```python
from build123d import *

# Parameters (mm, degrees)
ESQUISSE1_W             = 42
ESQUISSE1_H             = 42
BOSS_EXTRU_1_DEPTH      = 34
ESQUISSE2_R             = 11
BOSS_EXTRU_2_DEPTH      = 2
ESQUISSE3_R             = 2.5
BOSS_EXTRU_3_DEPTH      = 11.5
CHANFREIN1_SIZE         = 4
ESQUISSE4_W             = 17
ESQUISSE4_H             = 10
BOSS_EXTRU_4_DEPTH      = 5
ESQUISSE5_R             = 1.5
ENL_V_MAT_EXTRU_1_DEPTH = 5


with BuildPart() as part:
    # Esquisse1 → Boss.-Extru.1 (new body)
    with BuildSketch(Plane.XY):
        with Locations((21, 21)):
            Rectangle(ESQUISSE1_W, ESQUISSE1_H)
    extrude(amount=BOSS_EXTRU_1_DEPTH)

    # Esquisse2 → Boss.-Extru.2 (add)
    with BuildSketch(Plane.XY.offset(34)):
        with Locations((21, 21)):
            Circle(ESQUISSE2_R)
    extrude(amount=BOSS_EXTRU_2_DEPTH)

    # Esquisse3 → Boss.-Extru.3 (add)
    with BuildSketch(Plane.XY.offset(36)):
        with Locations((21, 21)):
            Circle(ESQUISSE3_R)
    extrude(amount=BOSS_EXTRU_3_DEPTH)

    # Chanfrein1
    chanfrein1_edges = [part.edges().sort_by_distance(p)[0] for p in [
        (0, 42, 17),
        (42, 42, 17),
        (42, 0, 17),
        (0, 0, 17),
    ]]
    chamfer(chanfrein1_edges, length=CHANFREIN1_SIZE)

    # Esquisse4 → Boss.-Extru.4 (add)
    with BuildSketch(Plane(origin=(0, 42, 0), x_dir=(1, 0, 0), z_dir=(0, 1, 0))):
        with Locations((21, -5)):
            Rectangle(ESQUISSE4_W, ESQUISSE4_H)
    extrude(amount=BOSS_EXTRU_4_DEPTH)

    # Esquisse5 → Enlèv. mat.-Extru.1 (cut)
    with BuildSketch(Plane.XY.offset(34)):
        with Locations((5.5, 36.5)):
            Circle(ESQUISSE5_R)
        with Locations((36.5, 36.5)):
            Circle(ESQUISSE5_R)
        with Locations((36.5, 5.5)):
            Circle(ESQUISSE5_R)
        with Locations((5.5, 5.5)):
            Circle(ESQUISSE5_R)
    extrude(amount=-ENL_V_MAT_EXTRU_1_DEPTH, mode=Mode.SUBTRACT)


solid = part.part
```
Design review of the part built by this model. Coordinates are the model's own, in mm. A direction names the side the tool comes from. Coordinates: 2 decimals unless noted, no trailing zeros. Loops run counter-clockwise (first coordinate to the right, second up) from the corner with the lowest first, then second, coordinate; pieces in that order, holes last. Notation, with made-up numbers: (-29, 5) - (12, 5) arc R15 ccw to (12, 27) - close; hole circle Ø3 at (-31, 73.5). An arc over 180 degrees is marked (long way). Use CSV: the item, a comma, the result in double quotes. Start each with the question number.
1) Consider section A-A on x = 21. Write out the cut boundary in (y, z), then the cut area to 3 significant figures.
2) Consider section D-D on y = 36.5. Write out the cut boundary in (x, z), then the cut area to 3 significant figures.
3) Tool access review of faces 1 (the flat face through (12.5, 44, 5)), 2 (the cylindrical face through (4.3, 4.6, 31.5)), 3 (the flat face through (29.5, 44, 5)), 4 (the flat face through (21, 44, 10)): name each direction out of +Z, -Z, +X, -X, +Y, -Y from which nothing blocks a thin tool from reaching the whole face with its end or side.
4) Consider section C-C on z = 28. Write out the cut boundary in (x, y), then the cut area to 3 significant figures.
5) Consider section B-B on y = 21. Write out the cut boundary in (x, z).
6) The part is to be moulded in two halves that separate along Y. For faces 5 (the flat face through (2, 2, 17)), 6 (the flat face through (36, 37, 29)), 7 (the flat face through (2, 40, 17)), 8 (the flat face through (5, 37, 29)), say which applies: +Y half, -Y half, draft (parallel to the pull), parting line (faces both ways), or undercut.
7) Wall thickness on L1, parallel to Y at x = 36.5, z = 30.6; L2, parallel to Y at x = 5, z = 31: over which ranges is each line inside the solid? List them lowest first. Write a range as from..to.
8) For pin 1 Ø3.5 at (x, y) = (5.5, 37) entering from +Z; pin 2 Ø1 at (x, y) = (16.5, 16) entering from +Z; pin 3 Ø2.5 at (y, z) = (45.5, 3) entering from -X, all flat-tipped, find the tip position at first contact; note any pin that passes through.
Geometry says:
1,outline,"(0, 0) - (47, 0) - (47, 10) - (42, 10) - (42, 34) - (32, 34) - (32, 36) - (23.5, 36) - (23.5, 47.5) - (18.5, 47.5) - (18.5, 36) - (10, 36) - (10, 34) - (0, 34) - close"
1,area,"1,580 mm^2"
2,outline,"(0, 0) - (42, 0) - (42, 34) - (38, 34) - (38, 29) - (35, 29) - (35, 34) - (7, 34) - (7, 29) - (4, 29) - (4, 34) - (0, 34) - close"
2,area,"1,400 mm^2"
3,face 1,"+Z, -Z, -X, +Y"
3,face 2,"+Z"
3,face 3,"+Z, -Z, +X, +Y"
3,face 4,"+Z, +X, -X, +Y"
4,outline,"(0, 4) - (4, 0) - (38, 0) - (42, 4) - (42, 38) - (38, 42) - (4, 42) - (0, 38) - close"
4,area,"1,730 mm^2"
5,outline,"(0, 0) - (42, 0) - (42, 34) - (32, 34) - (32, 36) - (23.5, 36) - (23.5, 47.5) - (18.5, 47.5) - (18.5, 36) - (10, 36) - (10, 34) - (0, 34) - close"
6,face 5,"-Y half"
6,face 6,"undercut"
6,face 7,"+Y half"
6,face 8,"undercut"
7,L1,"0..4, 7..35, 38..42"
7,L2,"0..4.09, 6.91..35.09, 37.91..42"
8,pin 1,"z = 34"
8,pin 2,"z = 36"
8,pin 3,"x = 12.5"
